```python
from build123d import *

# Parameters (mm, degrees)
SKETCH1_R           = 17.653
BOSS_EXTRUDE1_DEPTH = 10.287
SKETCH3_R           = 23.749
SKETCH3_R_2         = 12.7
CUT_EXTRUDE2_DEPTH  = 7.1628


with BuildPart() as part:
    # Sketch1 → Boss-Extrude1 (new body)
    with BuildSketch(Plane(origin=(0, 0, 0), x_dir=(1, 0, 0), z_dir=(0, 1, 0))):
        Circle(SKETCH1_R)
        Polygon((0, 7.361677812), (-6.3754, 3.680838906), (-6.3754, -3.680838906), (0, -7.361677812), (6.3754, -3.680838906), (6.3754, 3.680838906), align=None, mode=Mode.SUBTRACT)
    extrude(amount=BOSS_EXTRUDE1_DEPTH)

    # Sketch3 → Cut-Extrude2 (cut)
    with BuildSketch(Plane(origin=(0, 10.287, 0), x_dir=(1, 0, 0), z_dir=(0, 1, 0))):
        Circle(SKETCH3_R)
        Circle(SKETCH3_R_2, mode=Mode.SUBTRACT)
    extrude(amount=-CUT_EXTRUDE2_DEPTH, mode=Mode.SUBTRACT)


solid = part.part
```
Input: part model. Units: mm. Frame: model coordinates. A direction names the side the tool comes from. Round coordinates to 2 decimals unless told otherwise and drop trailing zeros. Loops run counter-clockwise (first coordinate to the right, second up) from the corner with the lowest first, then second, coordinate; pieces in that order, holes last. Notation, with made-up numbers: (-30.5, 11.5) - (11.5, 11.5) arc R24 ccw to (11.5, 22.5) - close; hole circle Ø3 at (13.5, 40). An arc over 180 degrees is marked (long way). One line per item, written item: value. Start each with the question number.
(1) Section D-D, the plane z = -11. Return loops of the section in (x, y), plus the area to 3 significant figures.
(2) Section B-B, the plane y = 9.75. Return loops of the section in (x, z).
(3) Draft query along X for faces 1 (the flat face through (-3.232, 5.071, 5.495)), 2 (the flat face through (-3, 10.287, -6)), 3 (the cylindrical face through (-2.75, 6.76, 12.4)). Return one class per face: +X half, -X half, draft (parallel to the pull), parting line (faces both ways), or undercut.
(4) Contact query for flat-ended pins moving along their axis: P1, Ø2, axis at y = 7.5, z = -1.5, coming from the +X side; P2, Ø3.5, axis at y = 5, z = -1, coming from the -X side; P3, Ø1, axis at x = 0.5, y = 8.5, coming from the -Z side. Output: stop coordinate, or through.
(5) Section C-C, the plane x = 3.5. Return loops of the section in (y, z).
(6) Section A-A, the plane z = 0. Return loops of the section in (x, y), plus the area to 3 significant figures.
(7) Ray query, line 1 (X direction, y = 3.5, z = 0.5); line 2 (Y direction, x = -16, z = 3); line 3 (Z direction, x = 0, y = 9). Return the intervals inside material, ascending. Write a range as [from, to].
(8) Access query for faces 4 (the flat face through (8, 0, 0)), 5 (the flat face through (-6.375, 5, 0)), 6 (the flat face through (8, 3.124, 12)). Directions: +Z, -Z, +X, -X, +Y, -Y. A direction counts if a zero-diameter tool reaches every point of the face in a straight line with its end or side. Return the directions, or none.
Results below:
1. outline: (-13.81, 0) - (13.81, 0) - (13.81, 3.12) - (6.35, 3.12) - (6.35, 10.29) - (-6.35, 10.29) - (-6.35, 3.12) - (-13.81, 3.12) - close
1. area: 177 mm^2
2. outline: circle Ø25.4 at (0, 0); hole (-6.38, -3.68) - (0, -7.36) - (6.38, -3.68) - (6.38, 3.68) - (0, 7.36) - (-6.38, 3.68) - close
3. face 1: undercut
3. face 2: draft
3. face 3: parting line
4. P1: x = 12.69
4. P2: x = -12.7
4. P3: z = -12.7
5. outline: (0, -17.3) - (3.12, -17.3) - (3.12, -12.21) - (10.29, -12.21) - (10.29, -5.34) - (0, -5.34) - close; (0, 5.34) - (10.29, 5.34) - (10.29, 12.21) - (3.12, 12.21) - (3.12, 17.3) - (0, 17.3) - close
6. outline: (-17.65, 0) - (-6.38, 0) - (-6.38, 10.29) - (-12.7, 10.29) - (-12.7, 3.12) - (-17.65, 3.12) - close; (6.38, 0) - (17.65, 0) - (17.65, 3.12) - (12.7, 3.12) - (12.7, 10.29) - (6.38, 10.29) - close
6. area: 161 mm^2
7. line 1: [-12.69, -6.38], [6.38, 12.69]
7. line 2: [0, 3.12]
7. line 3: [-12.7, -7.36], [7.36, 12.7]
8. face 4: +Z, -Z, +X, -X, -Y
8. face 5: +Y, -Y
8. face 6: +Y
